The listing builds one solid part. Answer for the finished solid, in the listing's coordinates (mm). Coordinates: 2 decimals unless noted, no trailing zeros. Order: outer loops, then holes, each group sorted by start corner. A loop starts at its lowest first (then second) coordinate and runs counter-clockwise, first axis right, second up. Notation, with made-up numbers: (82, -33) -> (140, -33) arc R19 ccw to (140, -15) -> close; hole circle Ø4 at (0.25, -9). An arc over 180 degrees is marked (long way). Answer in a Markdown table with one row per item.
```python
from build123d import *

# Parameters (mm, degrees)
SKETCH1_W           = 21.1
SKETCH1_H           = 15.748
SKETCH1_R           = 1.55575
SKETCH1_R_2         = 0.508
BOSS_EXTRUDE1_DEPTH = 0.5715


with BuildPart() as part:
    # Sketch1 → Boss-Extrude1 (new body, symmetric)
    with BuildSketch(Plane(origin=(0, 0, 0), x_dir=(1, 0, 0), z_dir=(0, 1, 0))):
        Rectangle(SKETCH1_W, SKETCH1_H)
        with Locations((-7.75, -5.23875)):
            Circle(SKETCH1_R, mode=Mode.SUBTRACT)
        with Locations((7.75, -5.23875)):
            Circle(SKETCH1_R, mode=Mode.SUBTRACT)
        with Locations((-8.89, 6.731)):
            Circle(SKETCH1_R_2, mode=Mode.SUBTRACT)
        with Locations((-6.35, 6.731)):
            Circle(SKETCH1_R_2, mode=Mode.SUBTRACT)
        with Locations((-3.81, 6.731)):
            Circle(SKETCH1_R_2, mode=Mode.SUBTRACT)
        with Locations((-1.27, 6.731)):
            Circle(SKETCH1_R_2, mode=Mode.SUBTRACT)
        with Locations((1.27, 6.731)):
            Circle(SKETCH1_R_2, mode=Mode.SUBTRACT)
        with Locations((3.81, 6.731)):
            Circle(SKETCH1_R_2, mode=Mode.SUBTRACT)
        with Locations((6.35, 6.731)):
            Circle(SKETCH1_R_2, mode=Mode.SUBTRACT)
        with Locations((8.89, 6.731)):
            Circle(SKETCH1_R_2, mode=Mode.SUBTRACT)
    extrude(amount=BOSS_EXTRUDE1_DEPTH, both=True)


solid = part.part
```
(1) For a pull along X with two mould halves and no side action, classify faces 1 (the cylindrical face through (-9.398, -0.008, -6.753)), 2 (the flat face through (0, 0, -7.874)), 3 (the flat face through (10.55, 0, 0)), 4 (the cylindrical face through (-4.318, -0.008, -6.753)) as released by +X, released by -X, zero draft, split by the parting line, or undercut.
Check values:
| item | result |
|---|---|
| face 1 | undercut |
| face 2 | zero draft |
| face 3 | released by +X |
| face 4 | undercut |
(2) Flat-ended cylindrical pins translate along their axes: pin 1 (1.6 mm diameter, centred on x = -3.81, z = -6.731, fed in from +Y); pin 2 (0.8 mm diameter, centred on x = -1.27, z = -6.731, fed in from +Y). Find the tip coordinate at first contact, or state that the pin passes through.
Check values:
| item | result |
|---|---|
| pin 1 | y = 0.57 |
| pin 2 | through |
(3) A cutting plane is placed at B-B, the plane z = 4. Determine the outline of the cut face in (x, y).
Check values:
| item | result |
|---|---|
| outline | (-10.55, -0.57) -> (-8.69, -0.57) -> (-8.69, 0.57) -> (-10.55, 0.57) -> close; (-6.81, -0.57) -> (6.81, -0.57) -> (6.81, 0.57) -> (-6.81, 0.57) -> close; (8.69, -0.57) -> (10.55, -0.57) -> (10.55, 0.57) -> (8.69, 0.57) -> close |
(4) A cutting plane is placed at C-C, the plane y = -0.3. Count the separate pieces of the cut face and the enclosed holes in it, then the cut area to 3 significant figures.
Check values:
| item | result |
|---|---|
| separate pieces | 1 |
| enclosed holes | 10 |
| area | 311 mm² |
(5) Find the intervals of material crossed by line 1 along Z through (x, y) = (7.75, 0.35); line 2 along Z through (x, y) = (-3.81, 0); line 3 along X through (y, z) = (0.1, 6.5), in increasing order. Write a range as from..to.
Check values:
| item | result |
|---|---|
| line 1 | -7.87..3.68, 6.79..7.87 |
| line 2 | -7.87..-7.24, -6.22..7.87 |
| line 3 | -10.55..-8.66, -6.84..6.84, 8.66..10.55 |
(6) A cutting plane is placed at A-A, the plane x = -3.81. Determine the outline of the cut face in (y, z).
Check values:
| item | result |
|---|---|
| outline | (-0.57, -7.87) -> (0.57, -7.87) -> (0.57, -7.24) -> (-0.57, -7.24) -> close; (-0.57, -6.22) -> (0.57, -6.22) -> (0.57, 7.87) -> (-0.57, 7.87) -> close |
(7) A cutting plane is placed at D-D, the plane x = -8.75. Determine the outline of the cut face in (y, z), then the cut area to 3 significant figures.
Check values:
| item | result |
|---|---|
| outline | (-0.57, -7.87) -> (0.57, -7.87) -> (0.57, -7.22) -> (-0.57, -7.22) -> close; (-0.57, -6.24) -> (0.57, -6.24) -> (0.57, 4.05) -> (-0.57, 4.05) -> close; (-0.57, 6.43) -> (0.57, 6.43) -> (0.57, 7.87) -> (-0.57, 7.87) -> close |
| area | 14.2 mm² |
